CAD build for the part. Positions are in the model's coordinates, mm. Face numbers are marked on the shaded views. Coordinates: 2 decimals unless noted, no trailing zeros. Order: outer loops, then holes, each group sorted by start corner. A loop starts at its lowest first (then second) coordinate and runs counter-clockwise, first axis right, second up.
Autodesk Inventor part; units mm, degrees
ref_plane "YZ Plane" through (0, 0, 0) normal (1, 0, 0) x (0, 1, 0)
ref_plane "XZ Plane" through (0, 0, 0) normal (0, 1, 0) x (-1, 0, 0)
ref_plane "XY Plane" through (0, 0, 0) normal (0, 0, 1) x (1, 0, 0)
sketch "Sketch1" plane through (0, 0, 0) normal (0, 0, 1) x (1, 0, 0)
  arc A0 (0, 6.1) -> (-0.3, -6.0926) centre (0, 0) ccw
  line L0 (0, -10.4012) -> (0, 10.52)
  line L1 (-0.3, -6.0926) -> (-0.3, -9.0926)
  arc A1 (-3.3, -8.478) -> (-0.3, -9.0926) centre (0, 0) ccw
  arc A2 (0, 8.4) -> (-3.3, -7.3926) centre (0, 0.1589) ccw
  line L2 (-3.3, -7.3926) -> (-3.3, -8.478)
  line L3 (0, 8.4) -> (0, 6.1)
  arc A3 (0.3, -6.0926) -> (0, 6.1) centre (0, 0) ccw
  line L4 (0.3, -6.0926) -> (0.3, -9.0926)
  arc A4 (0.3, -9.0926) -> (3.3, -8.478) centre (0, 0) ccw
  arc A5 (3.3, -7.3926) -> (0, 8.4) centre (0, 0.1589) ccw
  line L5 (3.3, -7.3926) -> (3.3, -8.478)
  line L6 (0, 8.4) -> (0, 6.1)
  dimension "d0" = 12.2
  dimension "d11" = 3
  dimension "d21" = 0.3
  dimension "d22" = 3
  dimension "d25" = 2.3
  dimension "d26" = 1.3
extrude "Extrusion1" add sketch "Sketch1" along normal blind 1.3
sketch "Sketch3" plane through (0, 0, 1.3) normal (0, 0, 1) x (1, 0, 0)
  line L0 (-0.3, -6.0926) -> (-0.3, -9.0926)
  line L1 (0, -12.5911) -> (0, 11.8985)
  point P0 (-1.8, -7.5926)
  point P1 (1.8, -7.5926)
  dimension "d30" = 1.5
  dimension "d31" = 1.5
hole "Hole1" at (-1.8, -7.5926, 1.3) at (1.8, -7.5926, 1.3) direction (0, 0, -1) diameter 1.2 end through all
fillet "Fillet1" radius 0.7667 8 edges at (0.3, -6.0926, 0.65) (-0.3, -6.0926, 0.65) (0.3, -9.0926, 0.65) (3.3, -8.478, 0.65) (-3.3, -8.478, 0.65) (-3.3, -7.3926, 0.65) (-0.3, -9.0926, 0.65) (3.3, -7.3926, 0.65)
equation "\"d32\" = Diam5"
equation "\"d39\" = 0.333333 * b"
equation "\"d0\" = Dg"
equation "\"d11\" = ParA"
equation "\"d21\" = 0.1 * ParA"
equation "\"d22\" = ParA"
equation "\"d25\" = b"
equation "\"d26\" = ParJ"
equation "\"d27\" = tt"
equation "\"b\" = 2.3"
equation "\"Dg\" = 12.2"
equation "\"ParJ\" = 1.3"
equation "\"ParA\" = 3"
equation "\"tt\" = 1.3"
equation "\"Diam5\" = 1.2"
equation "\"TEMPLATE\" = 1.2345"
properties part number "ANSI B27.8M - 3DM1-3DM1-13" material "Steel, Mild"
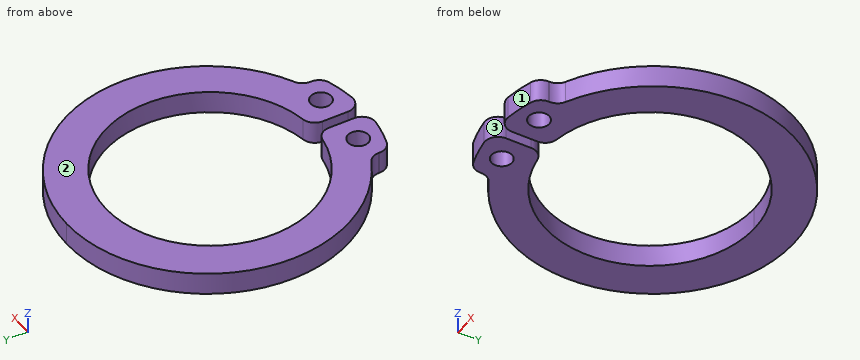
1) Slice it at D-D (x = -3.5). List the corners of the cut face in (y, z), plus the area to 3 significant figures.
2) Two-plate mould, pull along X, no slides. Class the marked faces 1, 2 and 3: released by +X, released by -X, zero draft, split by the parting line, or undercut.
3) Drill centre lines: probe 1 along Y at (x, z) = (1.8, 0.45); probe 2 along Y at (x, z) = (1.5, 1.15); probe 3 along X at (y, z) = (-6.25, 0.4). Where is each one in solid material? Low to high.
4) Slice it at A-A (z = 1.1). List the corners of the cut face in (x, y), plus the area to 3 significant figures.
5) Slice it at B-B (y = 0). List the corners of the cut face in (x, z), plus the area to 3 significant figures.
6) Pin check, flat tip, straight feed: P1, Ø4, axis at x = -6.5, y = 4, coming from the -Z side. Stop position of the tip, or through.
7) Slice it at C-C (x = -1.8). List the corners of the cut face in (y, z), plus the area to 3 significant figures.
Worked out:
1. outline: (-7.36, 0) - (-5, 0) - (-5, 1.3) - (-7.36, 1.3) - close; (5, 0) - (7.62, 0) - (7.62, 1.3) - (5, 1.3) - close
1. area: 6.49 mm2
2. face 1: released by +X
2. face 2: zero draft
2. face 3: undercut
3. probe 1: y = -8.92 to -8.19, -6.99 to -5.83, 5.83 to 8.2
3. probe 2: y = -8.97 to -8.11, -7.07 to -5.91, 5.91 to 8.26
3. probe 3: x = -5.18 to -0.52, 0.52 to 5.18
4. outline: (-3.72, -7.19) arc R0.77 cw to (-3.3, -7.88) - (-3.3, -7.94) arc R0.77 ccw to (-2.77, -8.67) arc R9.1 ccw to (-1.16, -9.02) arc R0.77 ccw to (-0.3, -8.26) - (-0.3, -6.78) arc R0.77 ccw to (-0.95, -6.03) arc R6.1 cw to (0, 6.1) arc R6.1 cw to (0.95, -6.03) arc R0.77 ccw to (0.3, -6.78) - (0.3, -8.26) arc R0.77 ccw to (1.16, -9.02) arc R9.1 ccw to (2.77, -8.67) arc R0.77 ccw to (3.3, -7.94) - (3.3, -7.88) arc R0.77 cw to (3.72, -7.19) arc R8.24 ccw to (0, 8.4) arc R8.24 ccw to start; hole circle Ø1.2 at (-1.8, -7.59); hole circle Ø1.2 at (1.8, -7.59)
4. area: 98.7 mm2
5. outline: (-8.24, 0) - (-6.1, 0) - (-6.1, 1.3) - (-8.24, 1.3) - close; (6.1, 0) - (8.24, 0) - (8.24, 1.3) - (6.1, 1.3) - close
5. area: 5.56 mm2
6. P1: stops at z = 0
7. outline: (-8.92, 0) - (-8.19, 0) - (-8.19, 1.3) - (-8.92, 1.3) - close; (-6.99, 0) - (-5.83, 0) - (-5.83, 1.3) - (-6.99, 1.3) - close; (5.83, 0) - (8.2, 0) - (8.2, 1.3) - (5.83, 1.3) - close
7. area: 5.54 mm2
